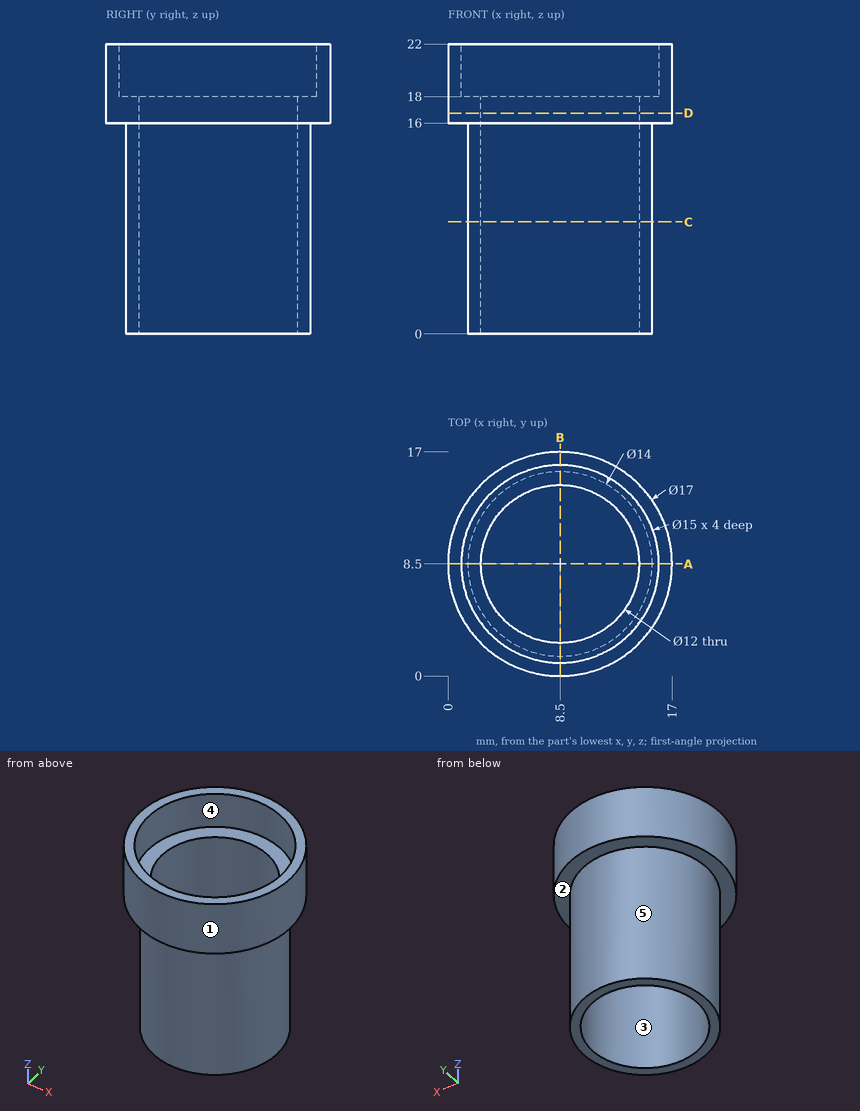
For this review, use the dimensioned drawing (mm, ordinates from the lowest corner) and the shaded views. A direction names the side the tool comes from. Round coordinates to 2 decimals unless told otherwise and drop trailing zeros. Order: outer loops, then holes, each group sorted by start corner. A loop starts at its lowest first (then second) coordinate and runs counter-clockwise, first axis right, second up. Notation, with made-up numbers: (49.5, 28.5) -> (69.5, 28.5) arc R25 cw to (69.5, 55.5) -> close; hole circle Ø8 at (38.5, -21). An arc over 180 degrees is marked (long way). Use CSV: the item, a comma, the result in double quotes. Start each with the question number.
(1) Consider section D-D on z = 16.75. Write out the cut boundary in (x, y).
(2) Mouldability with a two-part tool opening along Y and no side actions: class the marked faces 1, 2 and 3 as pulls with the +Y half, pulls with the -Y half, needs draft (parallel to the pull), parting line crosses it, or undercut.
(3) Consider section C-C on z = 8.5. Write out the cut boundary in (x, y).
(4) Insertion check: pin 1 (4 mm diameter, centred on x = 4.5, z = 15.5, fed in from -Y); pin 2 (8 mm diameter, centred on x = 12.5, z = 4, fed in from -Y); pin 3 (3 mm diameter, centred on x = 4, z = 13.5, fed in from -Y). Each pin has a flat end and moves straight along its axis. Give the tip position at first contact, or say it passes through.
(5) Wall thickness on probe 1 along Y at (x, z) = (8.5, 5); probe 2 along Y at (x, z) = (8.5, 19); probe 3 along Z at (x, y) = (10, 15): over which ranges is each line inside the solid? List them lowest first. Write a range as from..to.
(6) Consider section A-A on y = 8.5. Write out the cut boundary in (x, z), and give its area (3 significant figures).
(7) Tool access review of the marked faces 4 and 5: name each direction out of +Z, -Z, +X, -X, +Y, -Y from which nothing blocks a thin tool from reaching the whole face with its end or side.
Responses:
1,outline,"circle Ø17 at (8.5, 8.5); hole circle Ø12 at (8.5, 8.5)"
2,face 1,"parting line crosses it"
2,face 2,"needs draft"
2,face 3,"undercut"
3,outline,"circle Ø14 at (8.5, 8.5); hole circle Ø12 at (8.5, 8.5)"
4,pin 1,"y = 0.25"
4,pin 2,"y = 1.5"
4,pin 3,"y = 2.18"
5,probe 1,"1.5..2.5, 14.5..15.5"
5,probe 2,"0..1, 16..17"
5,probe 3,"0..18"
6,outline,"(0, 16) -> (1.5, 16) -> (1.5, 0) -> (2.5, 0) -> (2.5, 18) -> (1, 18) -> (1, 22) -> (0, 22) -> close; (14.5, 0) -> (15.5, 0) -> (15.5, 16) -> (17, 16) -> (17, 22) -> (16, 22) -> (16, 18) -> (14.5, 18) -> close"
6,area,"50.0 mm²"
7,face 4,"+Z"
7,face 5,"-Z"
